Can you work these out from the model? Positions are in its coordinate system, mm. A direction names the side the tool comes from. Round coordinates to 2 decimals unless told otherwise and drop trailing zeros. Loops run counter-clockwise (first coordinate to the right, second up) from the corner with the lowest first, then second, coordinate; pieces in that order, holes last.
from build123d import *

# Parameters (mm, degrees)
BOSS_EXTRUDE1_DEPTH = 457.2
SKETCH2_W           = 42.050956734
SKETCH2_H           = 23.599286926
CUT_EXTRUDE1_DEPTH  = 800
SKETCH3_W           = 114.4
SKETCH3_H           = 56.436670765
BOSS_EXTRUDE2_DEPTH = 10
SKETCH4_W           = 114.4
SKETCH4_H           = 4.244670765
CUT_EXTRUDE2_DEPTH  = 10
SKETCH7_W           = 48.1
SKETCH7_H           = 52.192
CUT_EXTRUDE3_DEPTH  = 42
SKETCH8_W           = 0.9
SKETCH8_H           = 40
CUT_EXTRUDE4_DEPTH  = 90
SPLIT1_START        = 342.8
SPLIT1_DEPTH        = 72.4
SPLIT1_START_2      = 19.95
SPLIT1_2_OUTLINE_W  = 52.192
SPLIT1_2_OUTLINE_H  = 72.4
SPLIT1_2_DEPTH      = 9.1
SPLIT1_START_3      = -19.05
SPLIT1_3_OUTLINE_W  = 17.78
SPLIT1_3_OUTLINE_H  = 72.4
SPLIT1_3_DEPTH      = 48.1
SPLIT1_4_OUTLINE_W  = 34.412
SPLIT1_4_OUTLINE_H  = 72.4
SPLIT1_4_DEPTH      = 9.1
SKETCH9_W           = 43.051140559
SKETCH9_H           = 19.836335545
CUT_EXTRUDE5_DEPTH  = 41
SKETCH10_W          = 39
SKETCH10_H          = 5.38616804
BOSS_EXTRUDE3_DEPTH = 47


# Read off the part's stored shape, not the designer's step: Split1
with BuildPart() as part:
    # Sketch1 → Boss-Extrude1 (new, symmetric)
    with BuildSketch(Plane.XY):
        Polygon((-19.05, 8.89), (19.05, 8.89), (19.05, 2.794), (3.81, 2.794), (3.81, -2.159), (9.779, -2.159), (9.779, -2.8321), (4.695818344, -8.89), (-4.695818344, -8.89), (-9.779, -2.8321), (-9.779, -2.159), (-3.81, -2.159), (-3.81, 2.794), (-19.05, 2.794), align=None)
    boss_extrude1 = extrude(amount=BOSS_EXTRUDE1_DEPTH, both=True)

    # Sketch2 → Cut-Extrude1 (cut)
    with BuildSketch(Plane(origin=(0, 0, -457.2), x_dir=(-1, 0, 0), z_dir=(0, 0, -1))):
        Rectangle(SKETCH2_W, SKETCH2_H)
    cut_extrude1 = extrude(amount=-CUT_EXTRUDE1_DEPTH, mode=Mode.SUBTRACT)

    # Sketch3 → Boss-Extrude2 (add)
    with BuildSketch(Plane(origin=(19.05, 0, 0), x_dir=(0, 0, -1), z_dir=(1, 0, 0))):
        with Locations((-400, -19.328335383)):
            Rectangle(SKETCH3_W, SKETCH3_H)
    extrude(amount=BOSS_EXTRUDE2_DEPTH)

    # Mirror1: Boss-Extrude1, Cut-Extrude1 across plane
    add(boss_extrude1.mirror(Plane(origin=(0, -17.206, 0), x_dir=(0, 0, 1), z_dir=(0, -1, 0))))
    add(cut_extrude1.mirror(Plane(origin=(0, -17.206, 0), x_dir=(0, 0, 1), z_dir=(0, -1, 0))), mode=Mode.SUBTRACT)

    # Sketch4 → Cut-Extrude2 (cut)
    with BuildSketch(Plane.ZY.offset(-19.05)):
        with Locations((400, -45.424335383)):
            Rectangle(SKETCH4_W, SKETCH4_H)
    extrude(amount=-CUT_EXTRUDE2_DEPTH, mode=Mode.SUBTRACT)

    # Sketch7 → Cut-Extrude3 (cut)
    with BuildSketch(Plane.XY.offset(457.2)):
        with Locations((5, -17.206)):
            Rectangle(SKETCH7_W, SKETCH7_H)
    extrude(amount=-CUT_EXTRUDE3_DEPTH, mode=Mode.SUBTRACT)

    # Sketch8 → Cut-Extrude4 (cut)
    with BuildSketch(Plane(origin=(0, 0, 342.8), x_dir=(-1, 0, 0), z_dir=(0, 0, -1))):
        with Locations((-19.5, -17.206)):
            Rectangle(SKETCH8_W, SKETCH8_H)
    extrude(amount=-CUT_EXTRUDE4_DEPTH, mode=Mode.SUBTRACT)

    # Split1 3 outline → Split1 3 (cut)
    with BuildSketch(Plane.YZ.offset(SPLIT1_START_3)):
        with Locations((0, 379)):
            Rectangle(SPLIT1_3_OUTLINE_W, SPLIT1_3_OUTLINE_H)
    extrude(amount=SPLIT1_3_DEPTH, mode=Mode.SUBTRACT)

    # Split1 4 outline → Split1 4 (cut)
    with BuildSketch(Plane.YZ.offset(SPLIT1_START_2)):
        with Locations((-26.096, 379)):
            Rectangle(SPLIT1_4_OUTLINE_W, SPLIT1_4_OUTLINE_H)
    extrude(amount=SPLIT1_4_DEPTH, mode=Mode.SUBTRACT)


with BuildPart() as body_2:
    # Split1 outline → Split1 (new body)
    with BuildSketch(Plane.XY.offset(SPLIT1_START)):
        Polygon((19.95, 2.794), (19.95, 8.89), (-19.05, 8.89), (-19.05, 2.794), (-3.81, 2.794), (-3.81, -2.159), (-9.779, -2.159), (-9.779, -2.8321), (-4.695818344, -8.89), (4.695818344, -8.89), (9.779, -2.8321), (9.779, -2.159), (3.81, -2.159), (3.81, 2.794), align=None)
    extrude(amount=SPLIT1_DEPTH)


with BuildPart() as body_3:
    # Split1 2 outline → Split1 2 (new body)
    with BuildSketch(Plane.YZ.offset(SPLIT1_START_2)):
        with Locations((-17.206, 379)):
            Rectangle(SPLIT1_2_OUTLINE_W, SPLIT1_2_OUTLINE_H)
    extrude(amount=SPLIT1_2_DEPTH)


with BuildPart() as part_1:
    add(part.part)

    # Combine1: cut body 3, body 2
    add(body_3.part, mode=Mode.SUBTRACT)
    add(body_2.part, mode=Mode.SUBTRACT)

    # Sketch9 → Cut-Extrude5 (cut)
    with BuildSketch(Plane.XY.offset(415.2)):
        with Locations((2.47557028, -33.383832228)):
            Rectangle(SKETCH9_W, SKETCH9_H)
    extrude(amount=-CUT_EXTRUDE5_DEPTH, mode=Mode.SUBTRACT)

    # Sketch10 → Boss-Extrude3 (add)
    with BuildSketch(Plane(origin=(0, -43.302, 0), x_dir=(-1, 0, 0), z_dir=(0, -1, 0))):
        with Locations((-0.45, -345.49308402)):
            Rectangle(SKETCH10_W, SKETCH10_H)
    extrude(amount=BOSS_EXTRUDE3_DEPTH)


solid = part_1.part
(1) If we section it at C-C, the plane y = -59: List the corners of the cut face in (x, z) for me, then the cut area to 3 significant figures.
Worked answers:
outline: (-19.05, 342.8) - (19.95, 342.8) - (19.95, 348.19) - (-19.05, 348.19) - close
area: 210 mm2
(2) If we section it at A-A, the plane z = 346: List the corners of the cut face in (x, y) for me.
Worked answers:
outline: (-19.05, -90.3) - (19.95, -90.3) - (19.95, -37.21) - (3.81, -37.21) - (3.81, -32.25) - (9.78, -32.25) - (9.78, -31.58) - (4.7, -25.52) - (-4.7, -25.52) - (-9.78, -31.58) - (-9.78, -32.25) - (-3.81, -32.25) - (-3.81, -37.21) - (-19.05, -37.21) - close
(3) Will these pins go through, and if not, where does the flat tip stop? P1, Ø0.7, axis at y = -32, z = 354.5, coming from the +X side; P2, Ø12, axis at x = -11, z = 366, coming from the +Y side; P3, Ø3, axis at x = 7.5, z = 362.5, coming from the -Y side.
Worked answers:
P1: stops at x = 9.78
P2: stops at y = -25.88
P3: stops at y = -43.3
(4) If I drill on line 1 (Z direction, x = -8.5, y = -87); line 2 (Y direction, x = -12, z = 367); line 3 (Y direction, x = 8, z = 366), over which ranges is the centre line in solid material (lowest first)?
Worked answers:
line 1: z = 342.8 to 348.19
line 2: y = -43.3 to -37.21
line 3: y = -43.3 to -37.21, -32.25 to -29.46
(5) If we section it at D-D, the plane x = 17: List the corners of the cut face in (y, z) for me, then the cut area to 3 significant figures.
Worked answers:
outline: (-90.3, 342.8) - (-37.21, 342.8) - (-37.21, 374.2) - (-43.3, 374.2) - (-43.3, 348.19) - (-90.3, 348.19) - close
area: 445 mm2
(6) If we section it at B-B, the plane x = -9: List the corners of the cut face in (y, z) for me.
Worked answers:
outline: (-90.3, 342.8) - (-37.21, 342.8) - (-37.21, 374.2) - (-43.3, 374.2) - (-43.3, 348.19) - (-90.3, 348.19) - close; (-32.25, 342.8) - (-30.65, 342.8) - (-30.65, 374.2) - (-32.25, 374.2) - close
(7) For faces 4 (the flat face through (3.81, -35, 359)), 5 (the flat face through (-11, -37.206, 359)), 6 (the flat face through (-7.202, -28.509, 358.72)), 7 (the flat face through (0, -43.302, 361)), 8 (the flat face through (7.27, -28.59, 358.72)), which set-ups out of +Z, -Z, +X, -X, +Y, -Y let a thin tool reach every point of the face, with its end or its side?
Worked answers:
face 4: +Z, -Z, +X
face 5: +Z, -Z, -X
face 6: +Z, -Z, -X, +Y
face 7: +Z, +X, -X, -Y
face 8: +Z, -Z, +X, +Y
(8) If we mould it in two halves opening along Y, with no side actions, what happens to faces 1 (the flat face through (0, -25.522, 359)), 2 (the flat face through (-19.05, -56, 348)), 3 (the flat face through (-7, -32.253, 359))? For each: released by +Y, released by -Y, zero draft, split by the parting line, or undercut.
Worked answers:
face 1: released by +Y
face 2: zero draft
face 3: undercut
